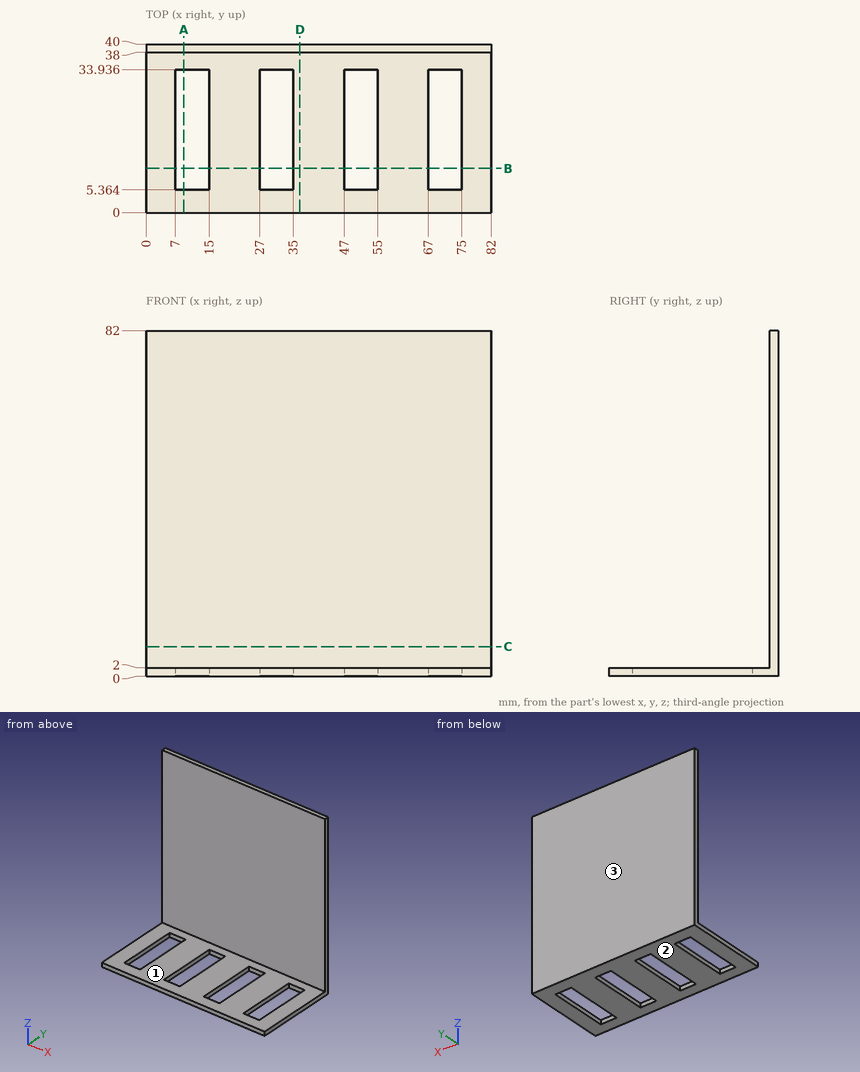
Study the drawing (mm; zero at the part's minimum x, y, z) and answer. Give positions to 0.01 mm unless a question says otherwise; leave off trailing zeros. Order: outer loops, then holes, each group sorted by start corner. A loop starts at its lowest first (then second) coordinate and runs counter-clockwise, first axis right, second up. Notation, with made-up numbers: (36.5, -28) - (87.5, -28) arc R24 cw to (87.5, -17) - close; hole circle Ø10 at (-9.75, -13.75). An arc over 180 degrees is marked (long way). Answer in a Markdown table with one row per item. Add a question column.
Q1. The part is cut by section D-D (x = 36.5). Determine the outline of the cut face in (y, z), then the cut area to 3 significant figures.
Q2. For a pull along Z with two mould halves and no side action, classify the marked faces 1, 2 and 3 as released by +Z, released by -Z, zero draft, split by the parting line, or undercut.
Q3. The part is cut by section C-C (z = 7). Determine the outline of the cut face in (x, y), then the cut area to 3 significant figures.
Q4. The part is cut by section B-B (y = 10.5). Determine the outline of the cut face in (x, z).
Q5. Given P1, Ø2, axis at x = 65.5, z = 46, coming from the -Y side; P2, Ø3, axis at x = 66, y = 13, coming from the +Z side, each flat-ended and moving along its own axis, determine where each tip first touches the part or whether it passes through.
Q6. Find the intervals of material crossed by line 1 along Y through (x, z) = (61.5, 78.5); line 2 along Z through (x, y) = (63.5, 23), in increasing order. Write a range as [from, to].
Q7. The part is cut by section A-A (x = 9). Determine the outline of the cut face in (y, z) (1 decimal), then the cut area to 3 significant figures.
Determined:
| question | item | result |
|---|---|---|
| 1 | outline | (0, 0) - (40, 0) - (40, 82) - (38, 82) - (38, 2) - (0, 2) - close |
| 1 | area | 240 mm² |
| 2 | face 1 | released by +Z |
| 2 | face 2 | released by -Z |
| 2 | face 3 | zero draft |
| 3 | outline | (0, 38) - (82, 38) - (82, 40) - (0, 40) - close |
| 3 | area | 164 mm² |
| 4 | outline | (0, 0) - (7, 0) - (7, 2) - (0, 2) - close; (15, 0) - (27, 0) - (27, 2) - (15, 2) - close; (35, 0) - (47, 0) - (47, 2) - (35, 2) - close; (55, 0) - (67, 0) - (67, 2) - (55, 2) - close; (75, 0) - (82, 0) - (82, 2) - (75, 2) - close |
| 5 | P1 | stops at y = 38 |
| 5 | P2 | stops at z = 2 |
| 6 | line 1 | y = [38, 40] |
| 6 | line 2 | z = [0, 2] |
| 7 | outline | (0, 0) - (5.4, 0) - (5.4, 2) - (0, 2) - close; (33.9, 0) - (40, 0) - (40, 82) - (38, 82) - (38, 2) - (33.9, 2) - close |
| 7 | area | 183 mm² |
